Autodesk Inventor part; units mm, degrees
ref_plane "Start Plane" through (0, 0, 110) normal (0, 0, 1) x (1, 0, 0)
ref_plane "End Plane" through (0, 0, 2000) normal (0, 0, 1) x (1, 0, 0)
ref_plane "Work Plane4" through (55, -1320, 110) normal (0, 0, -1) x (-1, 0, 0)
ref_plane "Start Plane" through (0, 0, 110) normal (0, 0, 1) x (1, 0, 0)
ref_plane "End Plane" through (0, 0, 2000) normal (0, 0, 1) x (1, 0, 0)
sketch "Sketch" plane through (0, 0, 0) normal (0, 0, 1) x (1, 0, 0)
  line L0 (-85, 167.3) -> (-22, 167.3)
  line L1 (-85, 180) -> (-85, 167.3)
  line L2 (85, 180) -> (-85, 180)
  line L3 (85, 167.3) -> (85, 180)
  line L4 (22, 167.3) -> (85, 167.3)
  line L5 (4, -149.3) -> (4, 149.3)
  line L6 (85, -167.3) -> (22, -167.3)
  line L7 (85, -180) -> (85, -167.3)
  line L8 (-85, -167.3) -> (-85, -180)
  line L9 (-22, -167.3) -> (-85, -167.3)
  line L10 (-4, 149.3) -> (-4, -149.3)
  line L11 (0, -252) -> (0, 252) construction
  line L12 (-4, -167.3) -> (4, -167.3) construction
  arc A0 (-22, -167.3) -> (-4, -149.3) centre (-22, -149.3) ccw
  arc A1 (-4, 149.3) -> (-22, 167.3) centre (-22, 149.3) ccw
  arc A2 (22, 167.3) -> (4, 149.3) centre (22, 149.3) ccw
  arc A3 (4, -149.3) -> (22, -167.3) centre (22, -149.3) ccw
  line L13 (-119, 0) -> (119, 0) construction
  line L14 (-85, -180) -> (85, -180)
  point P0 (-4, 167.3)
  point P1 (4, 167.3)
  point P2 (0, 0)
  point P3 (0, -167.3)
  point P4 (0, 0)
  dimension "d1" = 360
  dimension "d3" = 12.7
  dimension "d5" = 8
  dimension "d7" = 170
  dimension "d13" = 18
  dimension "d14" = 180
  dimension "d15" = 85
extrude "Body" add sketch "Sketch" along normal up to surface (1890 mm away) from surface at 110
sketch "Sketch3" plane through (0, 0, 0) normal (0, 0, 1) x (1, 0, 0)
  line L0 (0, 0) -> (10, 0)
ref_plane "Work Plane3" through (0, 0, 0) normal (0, -1, 0) x (1, 0, 0)
ref_plane "Work Plane4" through (55, -1320, 110) normal (0, 0, -1) x (-1, 0, 0)
split "Split1" plane through (55, -1320, 110) removes the side toward (0, 0, -1)
sketch "Sketch4" plane through (0, 0, 0) normal (0, -1, 0) x (1, 0, 0)
  line L0 (-2, 110) -> (12, 110)
  line L1 (-2, 2000) -> (12, 2000)
  dimension "d19" = 1890
equation "\"d1\" = ParH"
equation "\"d3\" = t2"
equation "\"d7\" = b"
equation "\"d13\" = R1"
equation "\"d14\" = 0.5 * d1"
equation "\"d15\" = 0.5 * d7"
equation "\"d8\" = G_L"
equation "\"b\" = 170"
equation "\"ParH\" = 360"
equation "\"R1\" = 18"
equation "\"G_L\" = d19"
equation "\"t1\" = 8"
equation "\"t2\" = 12.7"
equation "\"G_OFFSET_END\" = 0"
properties part number "DIN 1025 - IPE 360-1890" material "Steel, Mild"
Geometry check sheet. Reference: the model listing, model coordinates, mm. A direction names the side the tool comes from. Give positions to 0.01 mm unless a question says otherwise; leave off trailing zeros. Loops run counter-clockwise (first coordinate to the right, second up) from the corner with the lowest first, then second, coordinate; pieces in that order, holes last.
(1) Set-up check for faces 5 (the flat face through (53, 167.3, 1042)), 6 (the flat face through (0, 1, 2000)), 7 (the flat face through (-54, 167.3, 1042)): record each of +Z, -Z, +X, -X, +Y, -Y from which the full face is reachable in a straight line by a thin tool's end or side.
From the geometry:
face 5: +Z, -Z, +X
face 6: +Z, +X, -X, +Y, -Y
face 7: +Z, -Z, -X
(2) Section check C-C on y = -57.5. Record the cut outline in (x, z), then the cut area to 3 significant figures.
From the geometry:
outline: (-4, 110) - (4, 110) - (4, 2000) - (-4, 2000) - close
area: 15,100 mm2
(3) Section check B-B on z = 252.5. Record the cut outline in (x, y).
From the geometry:
outline: (-85, -180) - (85, -180) - (85, -167.3) - (22, -167.3) arc R18 cw to (4, -149.3) - (4, 149.3) arc R18 cw to (22, 167.3) - (85, 167.3) - (85, 180) - (-85, 180) - (-85, 167.3) - (-22, 167.3) arc R18 cw to (-4, 149.3) - (-4, -149.3) arc R18 cw to (-22, -167.3) - (-85, -167.3) - close
(4) Thickness scan on L1, parallel to Y at x = -78, z = 363.5; L2, parallel to X at y = 16, z = 429.5; L3, parallel to Y at x = 13, z = 424. Record the ranges inside material, lowest first.
From the geometry:
L1: y = -180 to -167.3, 167.3 to 180
L2: x = -4 to 4
L3: y = -180 to -164.89, 164.89 to 180
(5) Release check for a two-part mould opening along Y. For faces 1 (the flat face through (-4, 2, 1042)), 2 (the flat face through (1, 180, 1042)), 3 (the flat face through (-1, -180, 1042)), 4 (the flat face through (54, -167.3, 1042)) record: released by +Y, released by -Y, zero draft, split by the parting line, or undercut.
From the geometry:
face 1: undercut
face 2: released by +Y
face 3: released by -Y
face 4: undercut
(6) Depth check by flat-ended pin: pin 1 Ø6 at (y, z) = (87.5, 1721) entering from -X; pin 2 Ø1.5 at (y, z) = (124, 1738.5) entering from +X. Enter the tip coordinate at first touch or a pass-through.
From the geometry:
pin 1: stops at x = -4
pin 2: stops at x = 4
(7) Section check A-A on x = 41. Record the cut outline in (y, z), then the cut area to 3 significant figures.
From the geometry:
outline: (-180, 110) - (-167.3, 110) - (-167.3, 2000) - (-180, 2000) - close; (167.3, 110) - (180, 110) - (180, 2000) - (167.3, 2000) - close
area: 48,000 mm2
